The listing builds one solid part. Answer for the finished solid, in the listing's coordinates (mm). A direction names the side the tool comes from. Round coordinates to 2 decimals unless told otherwise and drop trailing zeros. Loops run counter-clockwise (first coordinate to the right, second up) from the corner with the lowest first, then second, coordinate; pieces in that order, holes last. Notation, with made-up numbers: (-35, -8) -> (22, -8) arc R20 ccw to (22, 22) -> close; hole circle Ø2 at (47.25, 57.5). An arc over 180 degrees is marked (long way). Answer in a Markdown table with one row per item. Add a question column.
```python
from build123d import *

# Parameters (mm, degrees)
SKETCH3_W           = 50
SKETCH3_H           = 50
SKETCH3_R           = 1.6
BOSS_EXTRUDE1_DEPTH = 4
BOSS_EXTRUDE3_DEPTH = 4
BOSS_EXTRUDE4_DEPTH = 3
BOSS_EXTRUDE5_DEPTH = 3


with BuildPart() as part:
    # Sketch3 → Boss-Extrude1 (new body)
    with BuildSketch(Plane(origin=(0, 0, 0), x_dir=(1, 0, 0), z_dir=(0, 1, 0))):
        with Locations((30.55, 30.55)):
            Rectangle(SKETCH3_W, SKETCH3_H)
        with Locations(Location((13.55, 47.55, 0), (0, 0, 270))):
            Circle(SKETCH3_R, mode=Mode.SUBTRACT)
        with Locations(Location((47.55, 47.55, 0), (0, 0, 270))):
            Circle(SKETCH3_R, mode=Mode.SUBTRACT)
        with Locations(Location((13.55, 13.55, 0), (0, 0, 270))):
            Circle(SKETCH3_R, mode=Mode.SUBTRACT)
        with Locations(Location((47.55, 13.55, 0), (0, 0, 270))):
            Circle(SKETCH3_R, mode=Mode.SUBTRACT)
    extrude(amount=BOSS_EXTRUDE1_DEPTH)

    # Sketch5 → Boss-Extrude3 (add)
    with BuildSketch(Plane(origin=(0, 0, -55.55), x_dir=(-1, 0, 0), z_dir=(0, 0, -1))):
        Polygon((-55.55, 4), (-55.55, 48.5), (-55.55, 55), (-46.05, 55), (-5.55, 55), (-5.55, 48.5), (-5.55, 5), (-5.55, 0), (-55.55, 0), align=None)
        with BuildLine():
            Line((-41.8, 33), (-41.8, 27))
            ThreePointArc((-41.8, 27), (-30.55, 15.75), (-19.3, 27))
            Line((-19.3, 27), (-19.3, 33))
            ThreePointArc((-19.3, 33), (-30.55, 44.25), (-41.8, 33))
        make_face(mode=Mode.SUBTRACT)
        with BuildLine():
            Line((-47.6, 48.5), (-47.6, 42.5))
            ThreePointArc((-47.6, 42.5), (-46.05, 40.95), (-44.5, 42.5))
            Line((-44.5, 42.5), (-44.5, 48.5))
            ThreePointArc((-44.5, 48.5), (-46.05, 50.05), (-47.6, 48.5))
        make_face(mode=Mode.SUBTRACT)
        with BuildLine():
            Line((-16.6, 48.5), (-16.6, 42.5))
            ThreePointArc((-16.6, 42.5), (-15.05, 40.95), (-13.5, 42.5))
            Line((-13.5, 42.5), (-13.5, 48.5))
            ThreePointArc((-13.5, 48.5), (-15.05, 50.05), (-16.6, 48.5))
        make_face(mode=Mode.SUBTRACT)
        with BuildLine():
            Line((-16.6, 17.5), (-16.6, 11.5))
            ThreePointArc((-16.6, 11.5), (-15.05, 9.95), (-13.5, 11.5))
            Line((-13.5, 11.5), (-13.5, 17.5))
            ThreePointArc((-13.5, 17.5), (-15.05, 19.05), (-16.6, 17.5))
        make_face(mode=Mode.SUBTRACT)
        with BuildLine():
            Line((-47.6, 17.5), (-47.6, 11.5))
            ThreePointArc((-47.6, 11.5), (-46.05, 9.95), (-44.5, 11.5))
            Line((-44.5, 11.5), (-44.5, 17.5))
            ThreePointArc((-44.5, 17.5), (-46.05, 19.05), (-47.6, 17.5))
        make_face(mode=Mode.SUBTRACT)
    extrude(amount=BOSS_EXTRUDE3_DEPTH)

    # Sketch7 → Boss-Extrude4 (add)
    with BuildSketch(Plane(origin=(55.55, 0, 0), x_dir=(0, 0, -1), z_dir=(1, 0, 0))):
        Polygon((55.55, 55), (5.55, 4), (55.55, 4), align=None)
    extrude(amount=-BOSS_EXTRUDE4_DEPTH)

    # Sketch8 → Boss-Extrude5 (add)
    with BuildSketch(Plane.ZY.offset(-5.55)):
        Polygon((-55.55, 55), (-5.55, 4), (-55.55, 4), align=None)
    extrude(amount=-BOSS_EXTRUDE5_DEPTH)


solid = part.part
```
Item 1: Section B-B, the plane x = 30.55 is taken. Write down the section's boundary in (y, z).
Item 2: The mould has two halves that part along Y. Classify faces 1 (the flat face through (52.55, 19, -41)), 2 (the cylindrical face through (30.303, 44.247, -57.522)), 3 (the cylindrical face through (46.08, 40.95, -57.52)), 4 (the flat face through (30, 55, -58)): +Y half, -Y half, draft (parallel to the pull), parting line (faces both ways), or undercut.
Item 3: For faces 5 (the flat face through (13.5, 14, -58)), 6 (the flat face through (55.55, 22, -38)), 7 (the flat face through (30, 4, -31)), determine the directions among +Z, -Z, +X, -X, +Y, -Y from which every point of the face is accessible in a straight line to the end or side of a thin tool.
Item 4: Section D-D, the plane y = 34 is taken. Write down the section's boundary in (x, z), and give its area (3 significant figures).
Item 5: Consider L1, parallel to X at y = 2.7, z = -13.55; L2, parallel to X at y = 33.5, z = -45. Determine where each line is inside the solid, lowest interval first. Write a range as from..to.
Item 6: Section C-C, the plane y = 46.5 is taken. Write down the section's boundary in (x, z), and give its area (3 significant figures).
Item 7: Section A-A, the plane z = -47.55 is taken. Write down the section's boundary in (x, y), and give its area (3 significant figures).
Item 8: Flat-ended cylindrical pins translate along their axes: P1, Ø3, axis at x = 46.5, y = 7, coming from the +Z side; P2, Ø2, axis at x = 30.5, z = -38.5, coming from the +Y side; P3, Ø2.5, axis at x = 13.55, z = -13.55, coming from the -Y side. Find the tip coordinate at first contact, or state that the pin passes through.
Here are the results:
| question | item | result |
|---|---|---|
| 1 | outline | (0, -59.55) -> (15.75, -59.55) -> (15.75, -55.55) -> (4, -55.55) -> (4, -5.55) -> (0, -5.55) -> close; (44.25, -59.55) -> (55, -59.55) -> (55, -55.55) -> (44.25, -55.55) -> close |
| 2 | face 1 | draft |
| 2 | face 2 | undercut |
| 2 | face 3 | undercut |
| 2 | face 4 | +Y half |
| 3 | face 5 | +Z, -Z |
| 3 | face 6 | +Z, -Z, +X, +Y, -Y |
| 3 | face 7 | +Z, +Y |
| 4 | outline | (5.55, -59.55) -> (19.34, -59.55) -> (19.34, -55.55) -> (8.55, -55.55) -> (8.55, -34.96) -> (5.55, -34.96) -> close; (41.76, -59.55) -> (55.55, -59.55) -> (55.55, -34.96) -> (52.55, -34.96) -> (52.55, -55.55) -> (41.76, -55.55) -> close |
| 4 | area | 234 mm² |
| 5 | L1 | x = 5.55..11.95, 15.15..45.95, 49.15..55.55 |
| 5 | L2 | x = 5.55..8.55, 52.55..55.55 |
| 6 | outline | (5.55, -59.55) -> (13.5, -59.55) -> (13.5, -55.55) -> (8.55, -55.55) -> (8.55, -47.22) -> (5.55, -47.22) -> close; (16.6, -59.55) -> (44.5, -59.55) -> (44.5, -55.55) -> (16.6, -55.55) -> close; (47.6, -59.55) -> (55.55, -59.55) -> (55.55, -47.22) -> (52.55, -47.22) -> (52.55, -55.55) -> (47.6, -55.55) -> close |
| 6 | area | 225 mm² |
| 7 | outline | (5.55, 0) -> (11.95, 0) -> (11.95, 4) -> (8.55, 4) -> (8.55, 46.84) -> (5.55, 46.84) -> close; (15.15, 0) -> (45.95, 0) -> (45.95, 4) -> (15.15, 4) -> close; (49.15, 0) -> (55.55, 0) -> (55.55, 46.84) -> (52.55, 46.84) -> (52.55, 4) -> (49.15, 4) -> close |
| 7 | area | 431 mm² |
| 8 | P1 | stops at z = -55.55 |
| 8 | P2 | stops at y = 4 |
| 8 | P3 | passes through |
